from build123d import *

# Parameters (mm, degrees)
SKETCH1_R           = 90
BOSS_EXTRUDE1_DEPTH = 30
SKETCH2_R           = 6.35
CUT_EXTRUDE2_DEPTH  = 131.766968306
CUT_EXTRUDE3_DEPTH  = 30
CIRPATTERN1_COUNT   = 5


with BuildPart() as part:
    # Sketch1 → Boss-Extrude1 (new body)
    with BuildSketch(Plane(origin=(0, 0, 0), x_dir=(0, 0, -1), z_dir=(1, 0, 0))):
        Circle(SKETCH1_R)
    extrude(amount=BOSS_EXTRUDE1_DEPTH)

    # Sketch2 → Cut-Extrude2 (cut, through all)
    with BuildSketch(Plane.ZY):
        Circle(SKETCH2_R)
    extrude(amount=-CUT_EXTRUDE2_DEPTH, mode=Mode.SUBTRACT)

    # Sketch3 → Cut-Extrude3 (cut)
    with BuildSketch(Plane.ZY):
        with BuildLine():
            Line((-20, 0), (-75, 0))
            ThreePointArc((-75, 0), (-69.290964938, 28.701257427), (-53.033008589, 53.033008589))
            Line((-53.033008589, 53.033008589), (-14.142135624, 14.142135624))
            ThreePointArc((-14.142135624, 14.142135624), (-18.47759065, 7.653668647), (-20, 0))
        make_face()
    cut_extrude3 = extrude(amount=-CUT_EXTRUDE3_DEPTH, mode=Mode.SUBTRACT)

    # CirPattern1: Cut-Extrude3 ×5 about axis
    cirpattern1_axis = Axis((0, 0, 0), (1, 0, 0))
    for i in range(1, CIRPATTERN1_COUNT):
        add(cut_extrude3.rotate(cirpattern1_axis, i * 360 / CIRPATTERN1_COUNT), mode=Mode.SUBTRACT)


solid = part.part
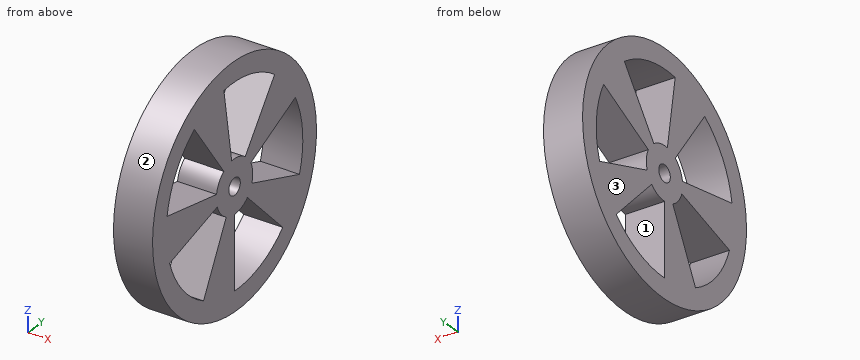
Can you work these out from the model? Positions are in its coordinate system, mm. Face numbers are marked on the shaded views. Round coordinates to 2 decimals unless told otherwise and drop trailing zeros. Loops run counter-clockwise (first coordinate to the right, second up) from the corner with the lowest first, then second, coordinate; pieces in that order, holes last. Notation, with made-up numbers: (79, 87.25) - (123, 87.25) arc R6 ccw to (123, 94.25) - close; hole circle Ø6 at (68.5, -5.75). An arc over 180 degrees is marked (long way). Use CSV: the item, a comma, the result in double quotes. Start each with the question number.
1) For pin 1 Ø4 at (x, y) = (18.5, -59) entering from -Z; pin 2 Ø2 at (x, y) = (6.5, -9) entering from -Z; pin 3 Ø6 at (x, y) = (21.5, -31.5) entering from +Z, each with a flat end and sliding along its axis, tell me the tip position at first contact or that it passes through.
2) If we section it at B-B on x = 13.5: Write out the boundary of the cut face in (y, z), plus the area to 3 significant figures.
3) If we section it at D-D on z = 65.5: Write out the boundary of the cut face in (x, y).
4) We'd pull the mould along Z, two halves only. Please class the marked faces 1, 2 and 3: released by +Z, released by -Z, zero draft, split by the parting line, or undercut.
5) If we section it at C-C on y = -30: Write out the boundary of the cut face in (x, z), plus the area to 3 significant figures.
6) If we section it at A-A on z = 0: Write out the boundary of the cut face in (x, y), plus the area to 3 significant figures.
7) Please list where these lines run through material, in increasing order: probe 1 along Y at (x, z) = (15, 0); probe 2 along Y at (x, z) = (22.25, -39); probe 3 along Z at (x, y) = (16.25, -43). Write a range as [from, to].
Geometry results:
1,pin 1,"stops at z = -69.65"
1,pin 2,"stops at z = -89.64"
1,pin 3,"stops at z = 85.37"
2,outline,"circle Ø180 at (0, 0); hole (-74.08, 11.73) - (-19.75, 3.13) arc R20 cw to (-11.76, 16.18) - (-44.08, 60.68) arc R75 ccw to start; hole (-71.33, -23.18) arc R75 ccw to (-34.05, -66.83) - (-9.08, -17.82) arc R20 cw to (-19.02, -6.18) - close; hole (-11.73, 74.08) - (-3.13, 19.75) arc R20 cw to (11.76, 16.18) - (44.08, 60.68) arc R75 ccw to start; hole circle Ø12.7 at (0, 0); hole (0, -75) arc R75 ccw to (53.03, -53.03) - (14.14, -14.14) arc R20 cw to (0, -20) - close; hole (17.82, 9.08) arc R20 cw to (19.02, -6.18) - (71.33, -23.18) arc R75 ccw to (66.83, 34.05) - close"
2,area,"15,100 mm2"
3,outline,"(0, -61.72) - (30, -61.72) - (30, -10.37) - (0, -10.37) - close; (0, 36.53) - (30, 36.53) - (30, 61.72) - (0, 61.72) - close"
4,face 1,"undercut"
4,face 2,"split by the parting line"
4,face 3,"zero draft"
5,outline,"(0, -84.85) - (30, -84.85) - (30, -58.88) - (0, -58.88) - close; (0, -9.75) - (30, -9.75) - (30, 4.75) - (0, 4.75) - close; (0, 41.29) - (30, 41.29) - (30, 84.85) - (0, 84.85) - close"
5,area,"2,520 mm2"
6,outline,"(0, -90) - (30, -90) - (30, -6.35) - (0, -6.35) - close; (0, 6.35) - (30, 6.35) - (30, 20) - (0, 20) - close; (0, 75) - (30, 75) - (30, 90) - (0, 90) - close"
6,area,"3,370 mm2"
7,probe 1,"y = [-90, -6.35], [6.35, 20], [75, 90]"
7,probe 2,"y = [-81.11, -64.06], [-19.87, 0], [39, 81.11]"
7,probe 3,"z = [-79.06, -61.45], [-13.97, 6.81], [59.18, 79.06]"
